Part model, mm, in its own coordinate system. A direction names the side the tool comes from. Round coordinates to 2 decimals unless told otherwise and drop trailing zeros. Write each loop counter-clockwise with the first axis right and the second up, starting at its lowest first coordinate (ties: lowest second). Pieces come first, ordered by that corner, then holes. Notation, with made-up numbers: M -13,36.5 L -9,36.5 A29 ccw -9,64.5 Z; hole C 62,45 d10. An arc over 180 degrees is marked long. Use one line per item in the form item = value. Start each with the question number.
Item 1: Cut at B-B, the plane x = -15.5. Give the cut face in (y, z), then the cut area to 3 significant figures.
Item 2: Mould opens along Z. For faces 1 (the face through (-30.373, 154.744, 130.946)), 2 (the face through (-30.472, 147.598, 129.899)), 3 (the face through (-32, 152, 134)), 4 (the face through (-33.7, 93.44, 85.62)) say: +Z half, -Z half, draft (parallel to the pull), parting line (faces both ways), or undercut.
Item 3: Probe L1, parallel to X at y = 201, z = 130.5; L2, parallel to X at y = 134.5, z = 88.5; L3, parallel to Z at x = 12, y = 188. List the from-to ranges inside material, lowest first.
Item 4: Flat gauge pins, fed straight in: pin 1 Ø5.5 at (y, z) = (149.5, 131) entering from +X; pin 2 Ø2 at (x, z) = (-21, -119.5) entering from +Y; pin 3 Ø1.5 at (y, z) = (140, -17.5) entering from -X. Where does each tip first touch, or does it go through?
Item 5: Cut at A-A, the plane x = 19. Give the cut face in (y, z).
Item 6: Which spindle directions (+Z, -Z, +X, -X, +Y, -Y) get a long thin tool onto all of the face, cutting with end or side? Do faces 5 (the face through (-37.399, 96, 82)), 6 (the face through (37.741, 98.67, 79.564)), 7 (the face through (-42.07, 94.82, 84.86)), 8 (the face through (-0.13, 181.52, 166.33)), 9 (the face through (38.866, 95.33, 85.329)). Say none if no direction does.
from build123d import *

# Parameters (mm, degrees)
REVOLUTION_ANGLE = 85
FILLET_R         = 8
PAD_DEPTH        = 8
POCKET_DEPTH     = 2
CHAMFER_SIZE     = 1
SKETCH005_W      = 3
SKETCH005_H      = 7
POCKET001_DEPTH  = 87.696576
POCKET002_DEPTH  = 78.501
SKETCH007_W      = 3
SKETCH007_H      = 6
POCKET003_DEPTH  = 87.696576


with BuildPart() as part:
    # Sketch → Revolution (revolve, symmetric)
    with BuildSketch(Plane.XY) as revolution_sk:
        with BuildLine():
            ThreePointArc((28, 223.38116), (0, 250), (-28, 223.38116))
            Line((-34.75, 90), (-28, 223.38116))
            Line((-34.75, 90), (-32.5, 90))
            Line((-32.5, 90), (-24.995207, 223.4))
            ThreePointArc((24.995207, 223.4), (0, 244.699412), (-24.995207, 223.4))
            Line((24.995207, 223.4), (32.5, 90))
            Line((32.5, 90), (34.75, 90))
            Line((34.75, 90), (28, 223.38116))
        make_face()
    revolve(axis=Axis((0, 0, 0), (1, 0, 0)), revolution_arc=REVOLUTION_ANGLE / 2)
    revolve(revolution_sk.sketch, axis=Axis((0, 0, 0), (-1, 0, 0)), revolution_arc=REVOLUTION_ANGLE / 2)

    # Fillet
    fillet_edges = [part.edges().sort_by_distance(p)[0] for p in [
        (33.625, 66.35496, 60.803119),
        (-33.625, 66.35496, 60.803119),
    ]]
    fillet(fillet_edges, radius=FILLET_R)

    # Sketch002 (on Face5 of Fillet) → Pad (new body)
    with BuildSketch(Plane(origin=(0, 0, 0), x_dir=(1, 0, 0), z_dir=(0, -0.67559, 0.737277))):
        Polygon((-43.394171, 132.697505), (-46.5, 121.106395), (-33.248819, 107.855214), (-31, 145.091677), align=None)
        Polygon((43.394171, 132.697505), (46.5, 121.106395), (33.248819, 107.855214), (31, 145.091677), align=None)
        Polygon((28, 194.106395), (32, 198.106395), (32, 206.106395), (28, 210.106395), (24, 206.106395), (24, 198.106395), align=None)
        Polygon((-28, 194.106395), (-24, 198.106395), (-24, 206.106395), (-28, 210.106395), (-32, 206.106395), (-32, 198.106395), align=None)
    extrude(amount=-PAD_DEPTH)

    # Sketch003 (on Face47 of Pad) → Pocket (cut)
    with BuildSketch(Plane(origin=(0, 0, 0), x_dir=(1, 0, 0), z_dir=(0, -0.67559, 0.737277))):
        Polygon((35, 146.869795), (45, 97.88), (47.939388, 98.48), (37.939388, 147.469795), align=None)
        Polygon((-47.939388, 98.48), (-45, 97.88), (-35, 146.869795), (-37.939388, 147.469795), align=None)
    extrude(amount=-POCKET_DEPTH, mode=Mode.SUBTRACT)

    # Chamfer
    chamfer_edges = [part.edges().sort_by_distance(p)[0] for p in [
        (42.094426, 93.718526, 85.877207),
        (38.89944, 94.199359, 86.317809),
        (-38.89944, 94.199359, 86.317809),
        (-42.094426, 93.718526, 85.877207),
    ]]
    chamfer(chamfer_edges, length=CHAMFER_SIZE)

    # Sketch005 (on Face6 of Chamfer) → Pocket001 (cut, through all)
    with BuildSketch(Plane(origin=(0, 5.404722, -5.898219), x_dir=(1, 0, 0), z_dir=(0, 0.67559, -0.737277))):
        with Locations((-36.047712, 125.078524)):
            Rectangle(SKETCH005_W, SKETCH005_H)
        with Locations((36.047712, 125.078524)):
            Rectangle(SKETCH005_W, SKETCH005_H)
    extrude(amount=-POCKET001_DEPTH, mode=Mode.SUBTRACT)

    # Sketch006 → Pocket002 (cut, through all)
    with BuildSketch(Plane.YZ.offset(32)):
        Polygon((154.311436, 128.180853), (156.149665, 125.810007), (160.891358, 129.486466), (159.053128, 131.857312), align=None)
    extrude(amount=-POCKET002_DEPTH, mode=Mode.SUBTRACT)

    # Sketch007 (on Face6 of Pocket002) → Pocket003 (cut, through all)
    with BuildSketch(Plane(origin=(0, 5.404722, -5.898219), x_dir=(1, 0, 0), z_dir=(0, 0.67559, -0.737277))):
        with Locations((-35.898523, -126.117473)):
            Rectangle(SKETCH007_W, SKETCH007_H)
        with Locations((35.898523, -126.117473)):
            Rectangle(SKETCH007_W, SKETCH007_H)
    extrude(amount=-POCKET003_DEPTH, mode=Mode.SUBTRACT)


solid = part.part
Model answer:
q1.outline = M 176.5,-161.74 L 180.87,-165.74 A245.33 ccw 180.87,165.74 L 176.5,161.74 A239.4 cw Z
q1.area = 2,130 mm²
q2.face_1 = undercut
q2.face_2 = undercut
q2.face_3 = draft
q2.face_4 = +Z half
q3.L1 = -21.76 to -15.17, 15.17 to 21.76
q3.L2 = -31.16 to -28.51, 28.51 to 31.16
q3.L3 = -160.67 to -151.86, 151.86 to 160.67
q4.pin_1 = 32
q4.pin_2 = 210.12
q4.pin_3 = -32.2
q5.outline = M 174.08,-159.52 L 178.85,-163.88 A242.58 ccw 178.85,163.88 L 174.08,159.52 A236.11 cw Z
q6.face_5 = none
q6.face_6 = +X, +Y
q6.face_7 = -Y
q6.face_8 = +Z, +X, -X, -Y
q6.face_9 = +Z
